Work out the finished part from the listing and answer in its coordinate system (mm). Round coordinates to 2 decimals unless told otherwise and drop trailing zeros. Order: outer loops, then holes, each group sorted by start corner. A loop starts at its lowest first (then second) coordinate and runs counter-clockwise, first axis right, second up. Notation, with made-up numbers: (-8.75, -29) -> (46.25, -29) arc R35 ccw to (46.25, 6) -> close; hole circle Ø11 at (-5.75, 15.25). An arc over 180 degrees is marked (long way). Use one line per item in the form item = value.
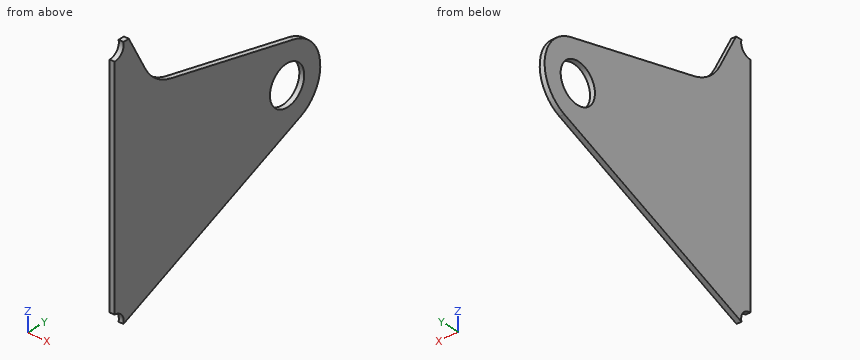
```python
from build123d import *

# Parameters (mm, degrees)
SKETCH_1_R           = 16
EXTRUDE_1_DEPTH      = 2
EXTRUDE_1_DEPTH_BACK = 2


with BuildPart() as part:
    # Sketch 1 → Extrude 1 (new body, two sides)
    with BuildSketch(Plane(origin=(0, 0, 0), x_dir=(0, 0, -1), z_dir=(1, 0, 0))) as extrude_1_sk:
        with BuildLine():
            Line((-91.5, -161), (91.5, -161))
            ThreePointArc((91.5, -161), (94.74405099, -154.319805392), (102, -152.738644179))
            Line((102, -152.738644179), (28.315921349, 12.617788956))
            ThreePointArc((28.315921349, 12.617788956), (-3.187422672, 30.835699063), (-30.298183379, 6.55896973))
            Line((-30.298183379, 6.55896973), (-55.212875562, -108.530738505))
            ThreePointArc((-55.212875562, -108.530738505), (-61.600879697, -122.455675592), (-73.25038996, -132.405518825))
            Line((-73.25038996, -132.405518825), (-102, -147.738644179))
            Line((-102, -147.738644179), (-102, -152.738644179))
            ThreePointArc((-102, -152.738644179), (-94.74405099, -154.319805392), (-91.5, -161))
        make_face()
        Circle(SKETCH_1_R, mode=Mode.SUBTRACT)
    extrude(amount=EXTRUDE_1_DEPTH)
    extrude(extrude_1_sk.sketch, amount=-EXTRUDE_1_DEPTH_BACK)


solid = part.part
```
Item 1: The part is cut by section A-A, the plane z = 0. Give the vertices of the cut face in (x, y), and give its area (3 significant figures).
Findings:
outline = (-2, -161) -> (2, -161) -> (2, -16) -> (-2, -16) -> close; (-2, 16) -> (2, 16) -> (2, 31) -> (-2, 31) -> close
area = 640 mm^2
Item 2: The part is cut by section D-D, the plane z = 41. Give the vertices of the cut face in (x, y), and give its area (3 significant figures).
Findings:
outline = (-2, -161) -> (2, -161) -> (2, -42.88) -> (-2, -42.88) -> close
area = 472 mm^2
Item 3: The part is cut by section B-B, the plane y = -2.5. Give the vertices of the cut face in (x, z), and give its area (3 significant figures).
Findings:
outline = (-2, -35.05) -> (2, -35.05) -> (2, -15.8) -> (-2, -15.8) -> close; (-2, 15.8) -> (2, 15.8) -> (2, 32.26) -> (-2, 32.26) -> close
area = 143 mm^2
Item 4: The part is cut by section C-C, the plane x = 1.2. Give the vertices of the cut face in (y, z).
Findings:
outline = (-161, -91.5) arc R8.5 cw to (-152.74, -102) -> (12.62, -28.32) arc R31 ccw to (6.56, 30.3) -> (-108.53, 55.21) arc R35.59 cw to (-132.41, 73.25) -> (-147.74, 102) -> (-152.74, 102) arc R8.5 cw to (-161, 91.5) -> close; hole circle Ø32 at (0, 0)
Item 5: A flat-ended cylindrical pin translates along its axis: P1, Ø1.5, axis at x = -1, z = -28, coming from the +Y side. Find the tip coordinate at first contact, or state that the pin passes through.
Findings:
P1 = 14.78
Item 6: Consider line 1 along Y through (x, z) = (-0.75, 0); line 2 along Z through (x, y) = (0.2, 3); line 3 along Z through (x, y) = (1.6, -12). Determine where each line is inside the solid, lowest interval first.
Findings:
line_1 = -161 to -16, 16 to 31
line_2 = -32.6 to -15.72, 15.72 to 31.07
line_3 = -39.29 to -10.58, 10.58 to 34.32
